```python
from build123d import *

# Parameters (mm, degrees)
SKETCH_3_W          = 93
SKETCH_3_H          = 60
EXTRUDE_1_DEPTH     = 6
SKETCH_6_W          = 93
SKETCH_6_H          = 80
EXTRUDE_3_DEPTH     = 8
SKETCH_7_W          = 76
SKETCH_7_H          = 10
CUT_EXTRUDE_1_DEPTH = 8
SKETCH_8_R          = 2
CUT_EXTRUDE_2_DEPTH = 8


with BuildPart() as part:
    # 草图3 → 凸台-拉伸1 (new body)
    with BuildSketch(Plane.XY):
        Rectangle(SKETCH_3_W, SKETCH_3_H)
    extrude(amount=EXTRUDE_1_DEPTH)

    # 草图6 → 凸台-拉伸3 (add)
    with BuildSketch(Plane.XY.offset(6)):
        Rectangle(SKETCH_6_W, SKETCH_6_H)
    extrude(amount=EXTRUDE_3_DEPTH)

    # 草图7 → 切除-拉伸1 (cut)
    with BuildSketch(Plane(origin=(0, 0, 6), x_dir=(-1, 0, 0), z_dir=(0, 0, -1))):
        with Locations((0, 35)):
            Rectangle(SKETCH_7_W, SKETCH_7_H)
        with Locations((0, -35)):
            Rectangle(SKETCH_7_W, SKETCH_7_H)
    extrude(amount=-CUT_EXTRUDE_1_DEPTH, mode=Mode.SUBTRACT)

    # 草图8 → 切除-拉伸2 (cut)
    with BuildSketch(Plane(origin=(0, 0, 6), x_dir=(-1, 0, 0), z_dir=(0, 0, -1))):
        with Locations((-42.5, 35)):
            Circle(SKETCH_8_R)
        with Locations(Location((42.5, 35, 0), (0, 0, 180))):
            Circle(SKETCH_8_R)
        with Locations((42.5, -35)):
            Circle(SKETCH_8_R)
        with Locations(Location((-42.5, -35, 0), (0, 0, 180))):
            Circle(SKETCH_8_R)
    extrude(amount=-CUT_EXTRUDE_2_DEPTH, mode=Mode.SUBTRACT)


solid = part.part
```
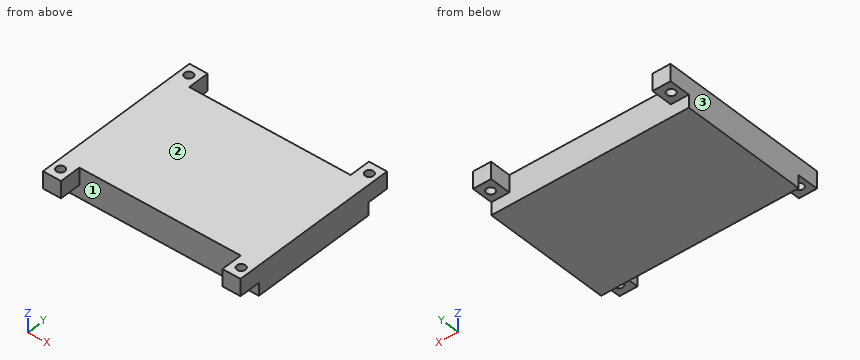
Read the model definition and answer for the solid it produces. Units are mm, in the model's axes. Face numbers are marked on the shaded views. Give positions to 0.01 mm unless a question says otherwise; leave off trailing zeros. Order: outer loops, then holes, each group sorted by start corner. A loop starts at its lowest first (then second) coordinate and runs counter-clockwise, first axis right, second up.
(1) Find section D-D (x = 13.5). Give the vertices of the cut face in (y, z).
(2) Find section C-C (z = 9.5). Give the vertices of the cut face in (x, y).
(3) Given pin 1 (3 mm diameter, centred on x = -42.5, y = 35, fed in from +Z); pin 2 (8 mm diameter, centred on x = 14, y = -5.5, fed in from -Z); pin 3 (1 mm diameter, centred on x = 7, z = 4, fed in from -Y); pin 4 (2.5 mm diameter, centred on x = 40.5, y = 33.5, fed in from -Z), each flat-ended and moving along its own axis, determine where each tip first touches the part or whether it passes through.
(4) Straight lines are drawn through the part: L1, parallel to Y at x = 42.5, z = 11.5; L2, parallel to X at y = 32, z = 6.5; L3, parallel to X at y = -36, z = 8.25. For each, find the intervals that lie inside material, in ascending order.
(5) Find section B-B (y = -35). Give the vertices of the cut face in (x, z), plus the area to 3 significant figures.
(6) Find section A-A (x = 42.5). Give the vertices of the cut face in (y, z).
(7) For a pull along X with two mould halves and no side action, classify the marked faces 1, 2 and 3 as released by +X, released by -X, zero draft, split by the parting line, or undercut.
Result sheet:
1. outline: (-30, 0) - (30, 0) - (30, 14) - (-30, 14) - close
2. outline: (-46.5, -40) - (-38, -40) - (-38, -30) - (38, -30) - (38, -40) - (46.5, -40) - (46.5, 40) - (38, 40) - (38, 30) - (-38, 30) - (-38, 40) - (-46.5, 40) - close; hole circle Ø4 at (-42.5, -35); hole circle Ø4 at (-42.5, 35); hole circle Ø4 at (42.5, -35); hole circle Ø4 at (42.5, 35)
3. pin 1: passes through
3. pin 2: stops at z = 0
3. pin 3: stops at y = -30
3. pin 4: stops at z = 6
4. L1: y = -40 to -37, -33 to 33, 37 to 40
4. L2: x = -46.5 to -38, 38 to 46.5
4. L3: x = -46.5 to -44.23, -40.77 to -38, 38 to 40.77, 44.23 to 46.5
5. outline: (-46.5, 6) - (-44.5, 6) - (-44.5, 14) - (-46.5, 14) - close; (-40.5, 6) - (-38, 6) - (-38, 14) - (-40.5, 14) - close; (38, 6) - (40.5, 6) - (40.5, 14) - (38, 14) - close; (44.5, 6) - (46.5, 6) - (46.5, 14) - (44.5, 14) - close
5. area: 72.0 mm2
6. outline: (-40, 6) - (-37, 6) - (-37, 14) - (-40, 14) - close; (-33, 6) - (-30, 6) - (-30, 0) - (30, 0) - (30, 6) - (33, 6) - (33, 14) - (-33, 14) - close; (37, 6) - (40, 6) - (40, 14) - (37, 14) - close
7. face 1: undercut
7. face 2: zero draft
7. face 3: released by -X
